Geometry: final body of the model. Coordinates: model frame, mm. Face numbers are marked on the shaded views. Give positions to 0.01 mm unless a question says otherwise; leave off trailing zeros. Loops run counter-clockwise (first coordinate to the right, second up) from the corner with the lowest first, then second, coordinate; pieces in that order, holes last.
from build123d import *

# Parameters (mm, degrees)
F0_W      = 140
F0_H      = 72.5
F1_DEPTH  = 8
F2_R      = 5
F4_R      = 6.784666
F5_DEPTH  = 0.5
F7_DEPTH  = 0.5
F5_FACE_R = 6.784666
F8_DEPTH  = 1
F9_W      = 3.526121
F9_H      = 21.039179
F10_DEPTH = 1
F11_W     = 11.203378
F11_H     = 2.960671
F12_DEPTH = 3
F13_R     = 1
F14_R     = 2.501655
F14_R_2   = 2.354917
F15_DEPTH = 3


with BuildPart() as f1:
    # F0 (on Top) → F1 (new body)
    with BuildSketch(Plane.XY):
        with Locations((2.468213, 9.830183)):
            Rectangle(F0_W, F0_H)
    extrude(amount=F1_DEPTH)

    # F2
    f2_edges = [f1.edges().sort_by_distance(p)[0] for p in [
        (72.468213, -26.419817, 4),
        (72.468213, 46.080183, 4),
        (-67.531787, -26.419817, 4),
        (-67.531787, 46.080183, 4),
    ]]
    fillet(f2_edges, radius=F2_R)

    # F4 (on face) → F5 (join)
    with BuildSketch(Plane.XY.offset(8)):
        with Locations((60.643088, 10.225745)):
            Circle(F4_R)
    extrude(amount=F5_DEPTH)

    # F6 (on face) → F7 (cut)
    with BuildSketch(Plane.XY.offset(8)):
        Polygon((49.707294, 42.785898), (-45.698922, 44.026859), (-45.698922, -21.970822), (49.707294, -21.970822), align=None)
    extrude(amount=-F7_DEPTH, mode=Mode.SUBTRACT)

    # F5_face (on face) → F8 (cut)
    with BuildSketch(Plane(origin=(60.643088, 10.225745, 8.5), x_dir=(1, 0, 0), z_dir=(0, 0, 1))):
        Circle(F5_FACE_R)
    extrude(amount=-F8_DEPTH, mode=Mode.SUBTRACT)

    # F9 (on face) → F10 (cut)
    with BuildSketch(Plane.XY.offset(8)):
        with Locations((-58.063432, 10.51959)):
            Rectangle(F9_W, F9_H)
    extrude(amount=-F10_DEPTH, mode=Mode.SUBTRACT)

    # F11 (on face) → F12 (join)
    with BuildSketch(Plane(origin=(-67.531787, 0, 0), x_dir=(0, -1, 0), z_dir=(-1, 0, 0))):
        with Locations((-33.545699, 4.414106)):
            Rectangle(F11_W, F11_H)
    extrude(amount=F12_DEPTH)

    # F13
    f13_edges = [f1.edges().sort_by_distance(p)[0] for p in [
        (-70.531787, 27.94401, 4.414106),
        (-70.531787, 39.147388, 4.414106),
    ]]
    fillet(f13_edges, radius=F13_R)

    # F14 (on face) → F15 (join)
    with BuildSketch(Plane(origin=(0, 46.080183, 0), x_dir=(-1, 0, 0), z_dir=(0, 1, 0))):
        with Locations((45.177385, 4.408034)):
            Circle(F14_R)
        with Locations((36.282312, 4.408034)):
            Circle(F14_R_2)
    extrude(amount=F15_DEPTH)


solid = f1.part
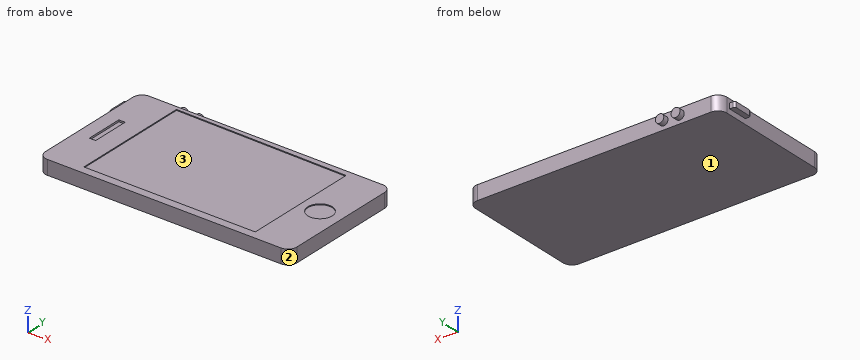
Item 1: Section query A-A on y = -18. Return loops of the section in (x, z).
Values follow:
outline: (-67.53, 0) - (72.47, 0) - (72.47, 8) - (49.71, 8) - (49.71, 7.5) - (-45.7, 7.5) - (-45.7, 8) - (-67.53, 8) - close
Item 2: Section query C-C on y = 5. Return loops of the section in (x, z).
Values follow:
outline: (-67.53, 0) - (72.47, 0) - (72.47, 8) - (64.97, 8) - (64.97, 7.5) - (56.32, 7.5) - (56.32, 8) - (49.71, 8) - (49.71, 7.5) - (-45.7, 7.5) - (-45.7, 8) - (-56.3, 8) - (-56.3, 7) - (-59.83, 7) - (-59.83, 8) - (-67.53, 8) - close
Item 3: Section query D-D on x = -50.5. Return loops of the section in (y, z), plus the area to 3 significant figures.
Values follow:
outline: (-26.42, 0) - (46.08, 0) - (46.08, 8) - (-26.42, 8) - close
area: 580 mm2
Item 4: Section query B-B on x = 3. Return loops of the section in (y, z).
Values follow:
outline: (-26.42, 0) - (46.08, 0) - (46.08, 8) - (43.39, 8) - (43.39, 7.5) - (-21.97, 7.5) - (-21.97, 8) - (-26.42, 8) - close
Item 5: Pin query (flat end, axial travel): pin 1 (5 mm diameter, centred on x = -45, y = -7, fed in from -Z); pin 2 (0.9 mm diameter, centred on x = -69, y = 31, fed in from -Z); pin 3 (1.5 mm diameter, centred on x = -68.5, y = 34.5, fed in from +Z); pin 4 (2 mm diameter, centred on x = 32.5, z = 3.5, fed in from +Y). Return the tip coordinate at first contact, or that it passes through.
Values follow:
pin 1: stops at z = 0
pin 2: stops at z = 2.93
pin 3: stops at z = 5.89
pin 4: stops at y = 46.08
Item 6: Draft query along X for the marked faces 1, 2 and 3. Return one class per face: +X half, -X half, draft (parallel to the pull), parting line (faces both ways), or undercut.
Values follow:
face 1: draft
face 2: +X half
face 3: undercut
Item 7: Ray query, probe 1 along X at (y, z) = (-7, 0.5); probe 2 along Y at (x, z) = (4.5, 1.75); probe 3 along Z at (x, y) = (6.5, -13.5). Return the intervals inside material, ascending.
Values follow:
probe 1: x = -67.53 to 72.47
probe 2: y = -26.42 to 46.08
probe 3: z = 0 to 7.5
